Print and shaded views of the part. All mm, measured from the part's lowest x, y and z. A direction names the side the tool comes from. Round coordinates to 2 decimals unless told otherwise and drop trailing zeros. Loops run counter-clockwise (first coordinate to the right, second up) from the corner with the lowest first, then second, coordinate; pieces in that order, holes last. Notation, with made-up numbers: (33.5, 4) - (45.5, 4) arc R25 ccw to (45.5, 36) - close; hole circle Ø2 at (88, -34). An arc over 180 degrees is marked (long way). Answer as a JSON object with one key per item and string values.
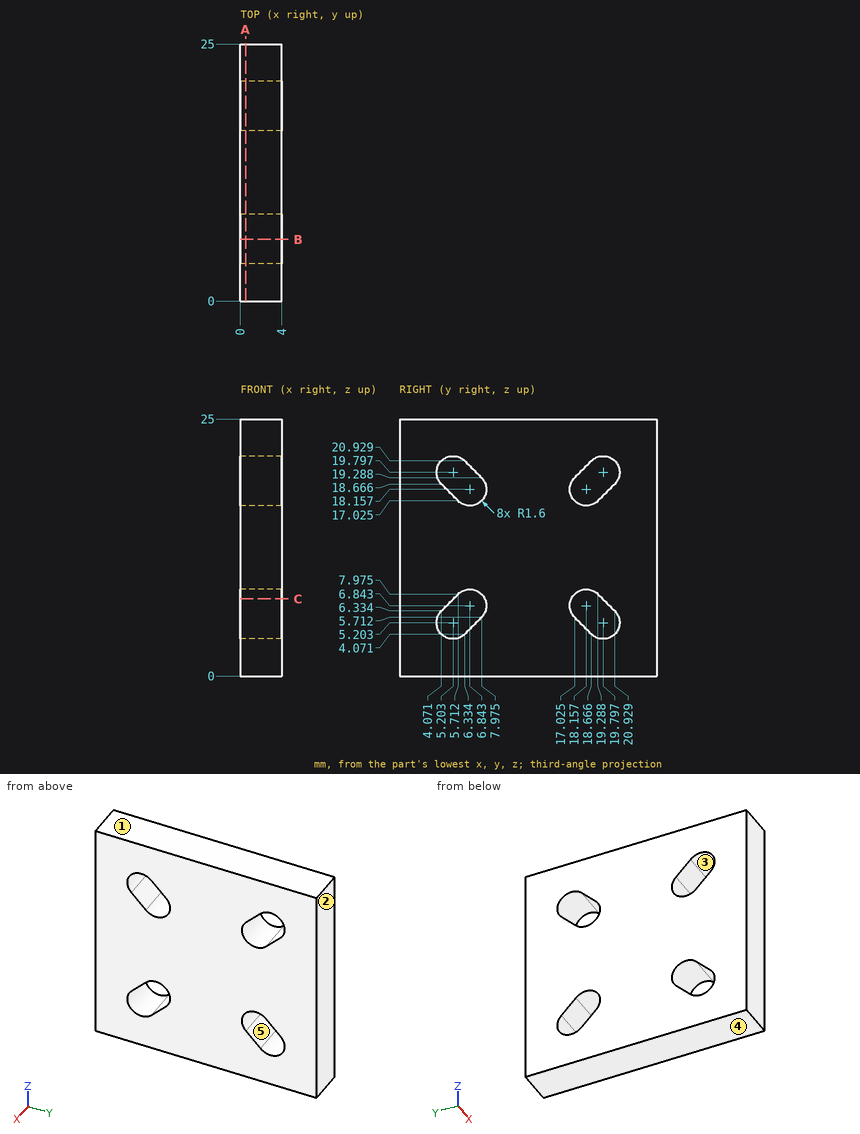
1) Probe probe 1 along Y at (x, z) = (2.45, 19) (1 decimal); probe 2 along Z at (x, y) = (1.55, 19.75) (1 decimal); probe 3 along Y at (x, z) = (1.05, 7.25) (1 decimal). List the from-to ranges inside material, lowest first.
Values follow:
{"probe 1": "0 to 3.8, 8.2 to 16.8, 21.2 to 25", "probe 2": "0 to 3.6, 7.5 to 17.5, 21.4 to 25", "probe 3": "0 to 5, 8.4 to 16.6, 20 to 25"}
2) Slice it at C-C on z = 7.5. List the corners of the cut face in (x, y).
Values follow:
{"outline": "(0, 0) - (4, 0) - (4, 5.24) - (0, 5.24) - close; (0, 8.3) - (4, 8.3) - (4, 16.7) - (0, 16.7) - close; (0, 19.76) - (4, 19.76) - (4, 25) - (0, 25) - close"}
3) Slice it at B-B on y = 6. List the corners of the cut face in (x, z) (1 decimal).
Values follow:
{"outline": "(0, 0) - (4, 0) - (4, 3.8) - (0, 3.8) - close; (0, 8.2) - (4, 8.2) - (4, 16.8) - (0, 16.8) - close; (0, 21.2) - (4, 21.2) - (4, 25) - (0, 25) - close"}
4) Tool access for the marked faces 4 and 5: list every direction of +Z, -Z, +X, -X, +Y, -Y with a clear straight run to the whole face (end or side of a thin tool).
Values follow:
{"face 4": "-Z, +X, -X, +Y, -Y", "face 5": "+X, -X"}
5) Slice it at A-A on x = 0.5. List the corners of the cut face in (y, z) (1 decimal), then the cut area to 3 significant figures.
Values follow:
{"outline": "(0, 0) - (25, 0) - (25, 25) - (0, 25) - close; hole (4.1, 6.3) arc R1.6 ccw to (6.3, 4.1) - (8, 5.7) arc R1.6 ccw to (5.7, 8) - close; hole (4.1, 18.7) - (5.7, 17) arc R1.6 ccw to (8, 19.3) - (6.3, 20.9) arc R1.6 ccw to start; hole (17, 5.7) - (18.7, 4.1) arc R1.6 ccw to (20.9, 6.3) - (19.3, 8) arc R1.6 ccw to start; hole (17, 19.3) arc R1.6 ccw to (19.3, 17) - (20.9, 18.7) arc R1.6 ccw to (18.7, 20.9) - close", "area": "563 mm²"}
6) Two-plate mould, pull along Y, no slides. Class the marked faces 1, 2 and 3: pulls with the +Y half, pulls with the -Y half, needs draft (parallel to the pull), parting line crosses it, or undercut.
Values follow:
{"face 1": "needs draft", "face 2": "pulls with the +Y half", "face 3": "undercut"}
